Part model, mm, in its own coordinate system. Face numbers are marked on the shaded views. A direction names the side the tool comes from. Give positions to 0.01 mm unless a question says otherwise; leave off trailing zeros. Loops run counter-clockwise (first coordinate to the right, second up) from the corner with the lowest first, then second, coordinate; pieces in that order, holes last. Notation, with made-up numbers: (53, 26) -> (58, 26) arc R31 ccw to (58, 53) -> close; hole circle Ø4 at (58.5, -34). An arc over 180 degrees is marked (long way). Write item = value, one per line.
Autodesk Inventor part; units mm, degrees
ref_plane "YZ Plane" through (0, 0, 0) normal (1, 0, 0) x (0, 1, 0)
ref_plane "XZ Plane" through (0, 0, 0) normal (0, 1, 0) x (-1, 0, 0)
ref_plane "XY Plane" through (0, 0, 0) normal (0, 0, 1) x (1, 0, 0)
sketch "Sketch1" plane through (0, 0, 0) normal (0, 1, 0) x (-1, 0, 0)
  circle A0 centre (0, 0) radius 7.5
  dimension "d0" = 15
extrude "Extrusion1" add sketch "Sketch1" along normal blind 3
sketch "Sketch2" plane through (0, 0, 0) normal (0, -1, 0) x (1, 0, 0)
  circle A0 centre (0, 0) radius 7.5
  circle A1 centre (0, 0) radius 2.3
  dimension "d3" = 4.6
extrude "Extrusion2" add sketch "Sketch2" along normal blind 3.2 contours A1
sketch "Sketch3" plane through (0, -3.2, 0) normal (0, -1, 0) x (1, 0, 0)
  circle A0 centre (0, 0) radius 2.3
  line L0 (-2.3, 5.3245) -> (-2.3, -5.3245)
  line L1 (2.3, 5.3245) -> (2.3, -5.3245)
  line L2 (0, 15.7328) -> (0, -15.032) construction
  circle A1 centre (0, 0) radius 7.5 construction
  arc A2 (-3, 6.8739) -> (-3, -6.8739) centre (0, 0) ccw construction
  arc A3 (3, -6.8739) -> (3, 6.8739) centre (0, 0) ccw construction
  arc A4 (2.3, 5.3245) -> (-2.3, 5.3245) centre (0, 0) ccw
  arc A5 (-2.3, -5.3245) -> (2.3, -5.3245) centre (0, 0) ccw
  dimension "d13" = 5.8
  dimension "d19" = 5.8
extrude "Extrusion3" add sketch "Sketch3" along normal blind 2.8
fillet "Fillet2" radius 1.2 4 edges at (-2.3, -4.6, 5.3245) (2.3, -4.6, 5.3245) (-2.3, -4.6, -5.3245) (2.3, -4.6, -5.3245)
ref_plane "Work Plane1" through (0, -3.2, 2.3) normal (1, 0, 0) x (0, 0, -1)
sketch "Sketch8" plane through (0, -3.2, 2.3) normal (1, 0, 0) x (0, 0, -1)
  line L0 (-3.5, -2.8) -> (26.5, -2.8) construction
  line L1 (-63.9924, 6.2) -> (53.0342, 6.2) construction
  line L2 (9.8, 3.2) -> (9.8, -146.8) construction
  arc A0 (9.8, 6.2) -> (4.3, 13.4284) centre (2.3, 6.2) ccw
  line L3 (-3.5, -2.8) -> (-3.0245, -2.8)
  line L4 (4.3, 13.4284) -> (4.3, 6.2)
  line L5 (4.3, 6.2) -> (9.8, 6.2)
  line L6 (-5.2, 3.2) -> (9.8, 3.2)
  line L7 (2.3, 3.2) -> (9.8, 3.2) construction
  line L8 (2.3, 6.2) -> (4.3, 6.2)
  line L9 (4.3, 6.2) -> (4.3, 105.8714)
  line L10 (2.3, 106.2) -> (2.3, 6.2)
  line L11 (2.3, 3.2) -> (2.3, 202.2325) construction
  arc A1 (2.3, 93.7) -> (2.3, 106.2) centre (2.3, 99.95) ccw
  line L12 (2.3, 106.2) -> (2.3, 93.7) construction
  line L13 (4.3, 105.8714) -> (2.3, 106.2)
  line L14 (2.3, 106.2) -> (2.3, 93.7)
  line L15 (2.3, -217.6065) -> (2.3, 271.0391)
  point P0 (37.0288, 0)
  point P1 (-3.3317, -2.8)
  dimension "d54" = 30
  dimension "d58" = 9
  dimension "d61" = 150
  dimension "d64" = 0
  dimension "d65" = 2
  dimension "d66" = 100
  dimension "d68" = 7.5
  dimension "d70" = 6.25
revolve "Revolution4" add sketch "Sketch8" angle 360 about axis through (0, 3, 0) along (0, 1, 0)
equation "\"d0\" = HeadConnectorOuterSize"
equation "\"d1\" = EarConnectorHeight"
equation "\"d3\" = HeadConnectorWidth - HeadConnectorTolerance"
equation "\"d4\" = HeadConnectorOuterHeight + HeadConnectorTolerance"
equation "\"d13\" = 0.5 * HeadConnectorDiam - HeadConnectorTolerance"
equation "\"d19\" = 0.5 * HeadConnectorDiam - HeadConnectorTolerance"
equation "\"d10\" = HeadConnectorHeight - HeadConnectorTolerance"
equation "\"d20\" = 0.2 * HeadConnectorProportion"
equation "\"d58\" = HeadConnectorOuterHeight + HeadConnectorHeight + EarConnectorHeight"
equation "\"d65\" = 0.5 * EarWidth"
equation "\"d66\" = EarHeight"
equation "\"d68\" = 0.5 * HeadConnectorOuterSize"
equation "\"d70\" = 0.5 * EarBallSize"
equation "\"EarHeight\" = 100"
equation "\"EarWidth\" = 4"
equation "\"EarBallSize\" = 12.5"
properties part number "EarShapeET"
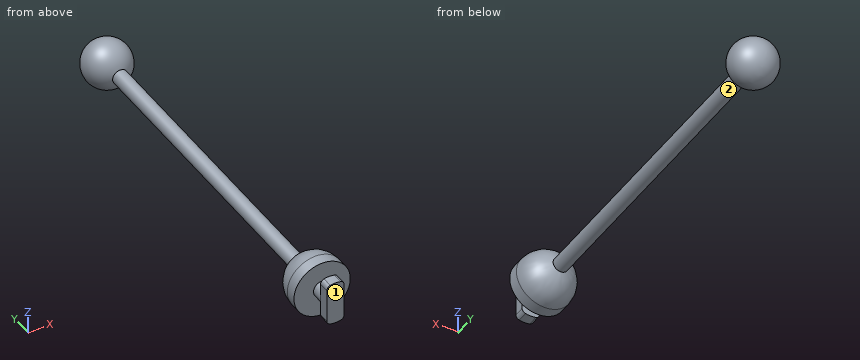
1) Which spindle directions (+Z, -Z, +X, -X, +Y, -Y) get a long thin tool onto all of the face, cutting with end or side? Do the marked faces 1 and 2. Say none if no direction does.
Resolved:
face_1 = +Z, -Z, +X, -X, -Y
face_2 = none
2) Slice it at A-A, the plane y = 44. List the corners of the cut face in (x, z), and give its area (3 significant figures).
Resolved:
outline = circle Ø4 at (0, 0)
area = 12.6 mm²
3) Drop flat-ended pins along their axis: P1, Ø3.5, axis at x = 1, z = -1.5, coming from the +Y side; P2, Ø5, axis at x = -3.5, y = 23, coming from the +Z side; P3, Ø1, axis at x = -1, y = 78, coming from the +Z side; P4, Ø3, axis at x = 3, y = 58, coming from the +Z side. Give the stop position or say it passes through.
Resolved:
P1 = 103
P2 = 1.73
P3 = 1.94
P4 = 1.32
4) Drill centre lines: line 1 along Y through (x, z) = (1.75, -3.5); line 2 along Y through (x, z) = (2, 3.5); line 3 along Y through (x, z) = (2.5, 1.75). Where is each one in solid material? Low to high. Write a range as [from, to].
Resolved:
line_1 = [-6, -3.2], [0, 9.4], [91.88, 101.62]
line_2 = [-6, -3.2], [0, 9.32], [91.97, 101.53]
line_3 = [0, 9.85], [91.3, 102.2]
